Work out the finished part from the listing and answer in its coordinate system (mm). A direction names the side the tool comes from. Give positions to 0.01 mm unless a question says otherwise; leave off trailing zeros. Write each loop counter-clockwise with the first axis right and the second up, starting at its lowest first coordinate (ties: lowest second). Pieces come first, ordered by that corner, then holes. Notation, with made-up numbers: (56.25, 15) -> (98.25, 15) arc R10 ccw to (98.25, 31) -> close; hole circle Ø6 at (-12.5, 43.25). An arc over 180 degrees is marked (long way). Write item = value, one per line. Start each with the question number.
from build123d import *

# Parameters (mm, degrees)
F0_W     = 10
F0_H     = 13
F1_DEPTH = 5
F2_T     = -1.2
F3_W     = 10
F3_H     = 5
F4_DEPTH = 2


with BuildPart() as f1:
    # F0 (on Top) → F1 (new body)
    with BuildSketch(Plane.XY):
        with Locations((2.011857, -5.49226)):
            Rectangle(F0_W, F0_H)
    extrude(amount=F1_DEPTH)

    # F2
    f2_openings = [f1.faces().sort_by_distance(p)[0] for p in [
        (2.011857, -11.99226, 2.5),
    ]]
    offset(amount=F2_T, openings=f2_openings)

    # F3 (on face) → F4 (join)
    with BuildSketch(Plane.XZ.offset(11.99226)):
        with Locations((2.011857, 2.5)):
            Rectangle(F3_W, F3_H)
    extrude(amount=F4_DEPTH)


solid = f1.part
(1) A cutting plane is placed at A-A, the plane y = -5.25. Write down the section's boundary in (x, z), then the cut area to 3 significant figures.
(2) A cutting plane is placed at B-B, the plane z = 3.05. Write down the section's boundary in (x, y), then the cut area to 3 significant figures.
(3) Find the intervals of material crossed by line 1 along Y through (x, z) = (2.5, 2.65); line 2 along X through (y, z) = (-6.5, 2.9); line 3 along Z through (x, y) = (-1.5, -10.75), in increasing order.
(4) For faces 4 (the flat face through (-1.788, -6, 2)), 5 (the flat face through (2, -6, 0)), determine the directions among +Z, -Z, +X, -X, +Y, -Y from which every point of the face is accessible in a straight line to the end or side of a thin tool.
(5) Determine the mould class of faces 1 (the flat face through (2, -13.992, 3)), 2 (the flat face through (2, -6, 1.2)), 3 (the flat face through (2, 1.008, 2)) for opening direction Y: pulls with the +Y half, pulls with the -Y half, needs draft (parallel to the pull), parting line crosses it, or undercut.
Results list:
q1.outline = (-2.99, 0) -> (7.01, 0) -> (7.01, 5) -> (-2.99, 5) -> close; hole (-1.79, 1.2) -> (5.81, 1.2) -> (5.81, 3.8) -> (-1.79, 3.8) -> close
q1.area = 30.2 mm²
q2.outline = (-2.99, -13.99) -> (7.01, -13.99) -> (7.01, 1.01) -> (-2.99, 1.01) -> close; hole (-1.79, -11.99) -> (5.81, -11.99) -> (5.81, -0.19) -> (-1.79, -0.19) -> close
q2.area = 60.3 mm²
q3.line_1 = -13.99 to -11.99, -0.19 to 1.01
q3.line_2 = -2.99 to -1.79, 5.81 to 7.01
q3.line_3 = 0 to 1.2, 3.8 to 5
q4.face_4 = none
q4.face_5 = -Z, +X, -X, +Y, -Y
q5.face_1 = pulls with the -Y half
q5.face_2 = undercut
q5.face_3 = pulls with the +Y half
